from build123d import *

# Parameters (mm, degrees)
SKETCH_1_R               = 25
EXTRUDE_1_DEPTH          = 2
SKETCH_2_R               = 7
CUT_EXTRUDE_2_DEPTH      = 3
SKETCH_3_R               = 2
CUT_EXTRUDE_3_DEPTH      = 3
PATTERN_CIRCULAR_1_COUNT = 4
CHAMFER_1_SIZE           = 1
CUT_EXTRUDE_START        = -3
CUT_EXTRUDE_4_DEPTH      = 3
PATTERN_CIRCULAR_3_COUNT = 16


with BuildPart() as part:
    # 草图1 → 拉伸1 (new body)
    with BuildSketch(Plane.XY):
        Circle(SKETCH_1_R)
    extrude(amount=EXTRUDE_1_DEPTH)

    # 草图2 → 拉伸2 (cut)
    with BuildSketch(Plane.XY.offset(2)):
        Circle(SKETCH_2_R)
    extrude(amount=-CUT_EXTRUDE_2_DEPTH, mode=Mode.SUBTRACT)

    # 草图3 → 拉伸3 (cut)
    with BuildSketch(Plane.XY.offset(2)):
        with Locations((-2.536174186, 12.750208645)):
            Circle(SKETCH_3_R)
    cut_extrude_3 = extrude(amount=-CUT_EXTRUDE_3_DEPTH, mode=Mode.SUBTRACT)

    # 阵列(圆周)1: 拉伸3 ×4 about axis
    pattern_circular_1_axis = Axis((0, 0, 0), (0, 0, 1))
    for i in range(1, PATTERN_CIRCULAR_1_COUNT):
        add(cut_extrude_3.rotate(pattern_circular_1_axis, i * 360 / PATTERN_CIRCULAR_1_COUNT), mode=Mode.SUBTRACT)

    # 倒角1
    chamfer_1_edges = [part.edges().sort_by_distance(p)[0] for p in [
        (-25, 0, 0),
    ]]
    chamfer(chamfer_1_edges, length=CHAMFER_1_SIZE)

    # 草图4 → 拉伸4 (cut)
    with BuildSketch(Plane.XY.offset(2).offset(CUT_EXTRUDE_START)):
        with BuildLine():
            Line((-18, 2.25), (-24.898544134, 2.25))
            ThreePointArc((-24.898544134, 2.25), (-25, 0), (-24.898544134, -2.25))
            Line((-24.898544134, -2.25), (-18, -2.25))
            ThreePointArc((-18, -2.25), (-15.75, 0), (-18, 2.25))
        make_face()
    cut_extrude_4 = extrude(amount=CUT_EXTRUDE_4_DEPTH, mode=Mode.SUBTRACT)

    # 阵列(圆周)3: 拉伸4 ×16 about axis
    pattern_circular_3_axis = Axis((0, 0, 0), (0, 0, 1))
    for i in range(1, PATTERN_CIRCULAR_3_COUNT):
        add(cut_extrude_4.rotate(pattern_circular_3_axis, i * 360 / PATTERN_CIRCULAR_3_COUNT), mode=Mode.SUBTRACT)


solid = part.part
Work out the finished part from the listing and answer in its coordinate system (mm). A direction names the side the tool comes from. Round coordinates to 2 decimals unless told otherwise and drop trailing zeros. Answer as CSV lines item,"result". Start each with the question number.
(1) The part is cut by section A-A, the plane y = 3. Give the number of separate pieces and of enclosed holes in the cut face, then the cut area to 3 significant figures.
(2) Find the intervals of material crossed by probe 1 along Y at (x, z) = (0, 0.65); probe 2 along Y at (x, z) = (1.5, 1.95); probe 3 along X at (y, z) = (4, 0.9), in increasing order.
(3) A tool of negligible diameter and unlimited length cuts with its end or side. For faces 1 (the flat face through (-10.305, 19, 0.986)), 2 (the flat face through (21, 2.25, 1)), 3 (the flat face through (13.61, 16.79, 0.99)), from which of +Z, -Z, +X, -X, +Y, -Y can it reach the whole face along a straight path? Write none if from no direction.
(4) Each of these flat-tipped pins is pushed along its axis until it touches: pin 1 (3.5 mm diameter, centred on x = 12.75, y = 2.54, fed in from +Z); pin 2 (8 mm diameter, centred on x = 19, y = -6.5, fed in from -Z); pin 3 (1 mm diameter, centred on y = 5.5, z = 0, fed in from -X); pin 4 (0.6 mm diameter, centred on y = 22, z = 1, fed in from -X). Where does it stop, or does it pass through?
(5) The mould has two halves that part along Y. Classify faces 4 (the cylindrical face through (-0.05, 15.75, 0.99)), 5 (the flat face through (2.25, -21, 1)), 6 (the flat face through (-6.148, -20.722, 0.986)), 7 (the flat face through (-10.27, -18.91, 0.99)): +Y half, -Y half, draft (parallel to the pull), parting line (faces both ways), or undercut.
Output values:
1,separate pieces,"3"
1,enclosed holes,"0"
1,area,"65.2 mm²"
2,probe 1,"y = -15.75 to -7, 7 to 15.75"
2,probe 2,"y = -16.32 to -14.46, -11.04 to -6.84, 6.84 to 16.32"
2,probe 3,"x = -24.58 to -5.74, 5.74 to 11.39, 14.11 to 24.58"
3,face 1,"+Z, -Z, +Y"
3,face 2,"+Z, -Z, +X"
3,face 3,"+Z, -Z"
4,pin 1,"passes through"
4,pin 2,"stops at z = 0"
4,pin 3,"stops at x = -23.89"
4,pin 4,"stops at x = -12.41"
5,face 4,"+Y half"
5,face 5,"draft"
5,face 6,"undercut"
5,face 7,"-Y half"
